from build123d import *

# Parameters (mm, degrees)
BOSS_EXTRUDE1_DEPTH = 80
SKETCH3_W           = 299
SKETCH3_H           = 299
BOSS_EXTRUDE2_DEPTH = 2
SKETCH4_W           = 82
SKETCH4_H           = 299
BOSS_EXTRUDE3_DEPTH = 2


with BuildPart() as part:
    # Sketch1 → Boss-Extrude1 (new body)
    with BuildSketch(Plane(origin=(0, 0, 0), x_dir=(0, 0, -1), z_dir=(1, 0, 0))):
        Polygon((-23.931657395, -26.597399746), (-23.931657395, 6.402600254), (9.068342605, 6.402600254), (9.068342605, 39.402600254), (42.068342605, 39.402600254), (42.068342605, 72.402600254), (75.068342605, 72.402600254), (75.068342605, 105.402600254), (108.068342605, 105.402600254), (108.068342605, 138.402600254), (141.068342605, 138.402600254), (141.068342605, 171.402600254), (174.068342605, 171.402600254), (174.068342605, 204.402600254), (207.068342605, 204.402600254), (207.068342605, 237.402600254), (240.068342605, 237.402600254), (240.068342605, 272.402600254), (238.068342605, 272.402600254), (238.068342605, 239.402600254), (205.068342605, 239.402600254), (205.068342605, 206.402600254), (172.068342605, 206.402600254), (172.068342605, 173.402600254), (139.068342605, 173.402600254), (139.068342605, 140.402600254), (106.068342605, 140.402600254), (106.068342605, 107.402600254), (73.068342605, 107.402600254), (73.068342605, 74.402600254), (40.068342605, 74.402600254), (40.068342605, 41.402600254), (7.068342605, 41.402600254), (7.068342605, 8.402600254), (-25.931657395, 8.402600254), (-25.931657395, -24.597399746), (-58.931657395, -24.597399746), (-58.931657395, -26.597399746), align=None)
    extrude(amount=BOSS_EXTRUDE1_DEPTH)

    # Sketch3 → Boss-Extrude2 (add)
    with BuildSketch(Plane.ZY):
        with Locations((-90.568342605, 122.902600254)):
            Rectangle(SKETCH3_W, SKETCH3_H)
    extrude(amount=BOSS_EXTRUDE2_DEPTH)

    # Sketch4 → Boss-Extrude3 (add)
    with BuildSketch(Plane.XZ.offset(26.597399746)):
        with Locations((39, -90.568342605)):
            Rectangle(SKETCH4_W, SKETCH4_H)
    extrude(amount=BOSS_EXTRUDE3_DEPTH)


solid = part.part
Geometry: final body of the model. Coordinates: model frame, mm. A direction names the side the tool comes from. Round coordinates to 2 decimals unless told otherwise and drop trailing zeros. Order: outer loops, then holes, each group sorted by start corner. A loop starts at its lowest first (then second) coordinate and runs counter-clockwise, first axis right, second up. Notation, with made-up numbers: (1.5, 6) -> (27.5, 6) arc R24 ccw to (27.5, 22) -> close; hole circle Ø6 at (88.5, 76.25). An arc over 180 degrees is marked (long way). Put each result on its own line as item: value. Start each with the question number.
Q1. Section A-A on z = -100. Return the cut outline in (x, y).
Q2. First-contact query: pin 1 (1 mm diameter, centred on x = 10, y = 38, fed in from +Z); pin 2 (6 mm diameter, centred on x = 42, z = -10.5, fed in from +Y); pin 3 (16.5 mm diameter, centred on x = 32, z = -56.5, fed in from +Y). Flat tips, straight axial feed; report the tip coordinate or a pass-through.
Q3. Reachability of faces 1 (the flat face through (30, 245, -240.068)), 2 (the flat face through (39, 8.403, 9)), 3 (the flat face through (39, 155, -141.068)) from +Z, -Z, +X, -X, +Y, -Y: full face, straight path, thin tool, end or side. Return the list, or none.
Q4. Pull-direction query (Y, two-part tool) for faces 4 (the flat face through (39, 223, -205.068)), 5 (the flat face through (-0.3, 272.403, -91.3)), 6 (the flat face through (39, 89, -75.068)); classes: +Y half, -Y half, draft (parallel to the pull), parting line (faces both ways), or undercut.
Q5. Section B-B on y = 112. Return the cut outline in (x, z).
Q6. Line query: probe 1 along Y at (x, z) = (75, 20.5); probe 2 along Y at (x, z) = (57, -121); probe 3 along Z at (x, y) = (14, 48.5). Output: solid intervals per line, ascending.
Ans:
1. outline: (-2, -28.6) -> (80, -28.6) -> (80, -26.6) -> (0, -26.6) -> (0, 105.4) -> (80, 105.4) -> (80, 107.4) -> (0, 107.4) -> (0, 272.4) -> (-2, 272.4) -> close
2. pin 1: stops at z = -7.07
2. pin 2: stops at y = 41.4
2. pin 3: stops at y = 74.4
3. face 1: -Z, +X, -X, +Y, -Y
3. face 2: +Z, +X, +Y
3. face 3: -Z, +X
4. face 4: draft
4. face 5: +Y half
4. face 6: undercut
5. outline: (-2, -240.07) -> (0, -240.07) -> (0, -108.07) -> (80, -108.07) -> (80, -106.07) -> (0, -106.07) -> (0, 58.93) -> (-2, 58.93) -> close
6. probe 1: y = -28.6 to -26.6, 6.4 to 8.4
6. probe 2: y = -28.6 to -26.6, 138.4 to 140.4
6. probe 3: z = -42.07 to -40.07
